Work out the finished part from the listing and answer in its coordinate system (mm). Give positions to 0.01 mm unless a question says otherwise; leave off trailing zeros. Write each loop counter-clockwise with the first axis right and the second up, starting at its lowest first coordinate (ties: lowest second). Pieces come first, ordered by that corner, then holes. Notation, with made-up numbers: (40, 75) -> (44, 75) arc R24 cw to (44, 109) -> close; hole circle Ø4 at (73, 56.5). An arc over 180 degrees is marked (long way). Use a Markdown table: item, result. Add a question column.
Q1. Consider line 1 (Z direction, x = 0, y = 8.25); line 2 (Y direction, x = -1.5, z = 1.2). Determine where each line is inside the solid, lowest interval first.
Q2. Section A-A, the plane y = 109 is taken. Give the vertices of the cut face in (x, z).
Q3. This flat-tipped pin is pushed along its axis until it touches: pin 1 Ø2 at (y, z) = (59, 1.5) entering from -X. Where does it stop, or does it pass through?
from build123d import *

# Parameters (mm, degrees)
ESBO_O1_R                     = 3
RESSALTO_EXTRUS_O1_DEPTH      = 135.5
FURO_ROSCADO_DE_M3X0_51_D     = 2.5
FURO_ROSCADO_DE_M3X0_51_DEPTH = 18.5
FURO_ROSCADO_DE_M3X0_51_TIP   = 0.751075774
ESBO_O10_R                    = 1.5
RESSALTO_EXTRUS_O2_DEPTH      = 5


with BuildPart() as part:
    # Esboço1 → Ressalto-extrusão1 (new body)
    with BuildSketch(Plane(origin=(0, 0, 0), x_dir=(1, 0, 0), z_dir=(0, 1, 0))):
        Circle(ESBO_O1_R)
    extrude(amount=RESSALTO_EXTRUS_O1_DEPTH)

    # Furo roscado de M3x0.51
    with Locations(Plane.XZ):
        with Locations((0, 0)):
            Hole(FURO_ROSCADO_DE_M3X0_51_D / 2, depth=FURO_ROSCADO_DE_M3X0_51_DEPTH)
            with Locations((0, 0, -(FURO_ROSCADO_DE_M3X0_51_DEPTH + FURO_ROSCADO_DE_M3X0_51_TIP / 2))):  # 118° drill point
                Cone(0, FURO_ROSCADO_DE_M3X0_51_D / 2, FURO_ROSCADO_DE_M3X0_51_TIP, mode=Mode.SUBTRACT)

    # Esboço10 → Ressalto-extrusão2 (add)
    with BuildSketch(Plane(origin=(0, 135.5, 0), x_dir=(1, 0, 0), z_dir=(0, 1, 0))):
        Circle(ESBO_O10_R)
    extrude(amount=RESSALTO_EXTRUS_O2_DEPTH)


solid = part.part
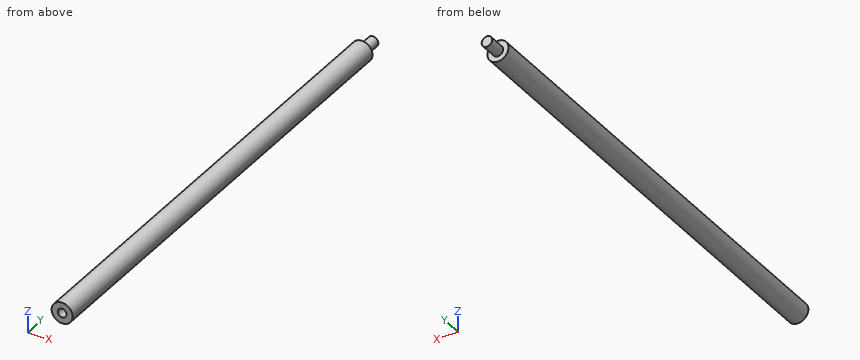
Result set:
| question | item | result |
|---|---|---|
| 1 | line 1 | z = -3 to -1.25, 1.25 to 3 |
| 1 | line 2 | y = 0 to 135.5 |
| 2 | outline | circle Ø6 at (0, 0) |
| 3 | pin 1 | stops at x = -2.96 |
